Could you check a few things on this drawing? It's one solid part, dimensions in mm from its lowest x, y, z. A direction names the side the tool comes from. Round coordinates to 2 decimals unless told otherwise and drop trailing zeros. Loops run counter-clockwise (first coordinate to the right, second up) from the corner with the lowest first, then second, coordinate; pieces in that order, holes last. Notation, with made-up numbers: M 10,75.5 L 66,75.5 A11 cw 66,91.5 Z; hole C -37,-34 d2. An arc over 180 degrees is marked long. Put each result on its own line as item: value. Start each with the question number.
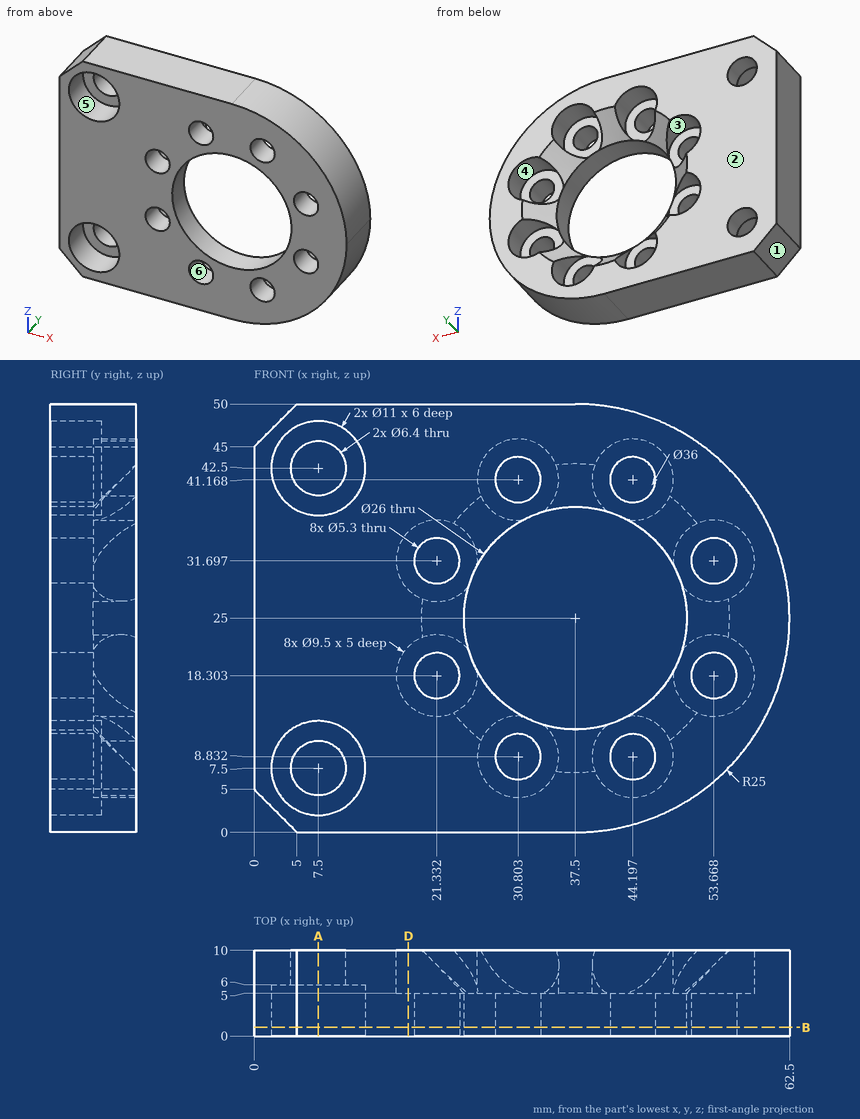
1) Suppose I cut it at B-B (y = 1). State how many separate pieces and enclosed holes the cut face has, plus the area to 3 significant figures.
2) If I drill on probe 1 along Z at (x, y) = (43.5, 4) (1 decimal); probe 2 along X at (y, z) = (1.25, 42); probe 3 along Z at (x, y) = (4.5, 4.75), over which ranges is the centre line in solid material (lowest first)? Write a range as from..to.
3) If we mould it in two halves opening along Z, with no side actions, what happens to the marked faces 1, 2 and 3? For each: pulls with the +Z half, pulls with the -Z half, needs draft (parallel to the pull), parting line crosses it, or undercut.
4) Suppose I cut it at D-D (x = 18). Write out the boundary of the cut face in (y, z).
5) On a 3-axis mill with a long thin cutter (end or side, diameter ignored), from which of +Z, -Z, +X, -X, +Y, -Y can I reach the whole of each face in a straight line? I mean the marked faces 4, 5 and 6. Say none if no direction works.
6) Suppose I cut it at A-A (x = 7.5). Write out the boundary of the cut face in (y, z).
7) I'm going to push flat-ended pins straight in: P1, Ø4.5, axis at x = 33, z = 8, coming from the +Y side; P2, Ø3, axis at x = 44.2, z = 41.17, coming from the +Y side; P3, Ø1.5, axis at y = 4, z = 37, coming from the +X side; P4, Ø1, axis at y = 3, z = 9.5, coming from the +X side. Where does each tip first touch, or does it pass through?
Results are:
1. separate pieces: 1
1. enclosed holes: 11
1. area: 1,930 mm²
2. probe 1: 0.7..6.3, 11.4..13.5, 36.5..38.6, 43.7..49.3
2. probe 2: 0..2.02, 12.98..28.29, 33.32..41.68, 46.71..55.83
2. probe 3: 0.5..2.89, 12.11..37.89, 47.11..49.5
3. face 1: pulls with the -Z half
3. face 2: needs draft
3. face 3: undercut
4. outline: M 0,0 L 10,0 L 10,14.92 L 5,14.92 L 5,21.69 L 10,21.69 L 10,28.31 L 5,28.31 L 5,35.08 L 10,35.08 L 10,50 L 0,50 Z
5. face 4: +Y
5. face 5: -Y
5. face 6: +Y, -Y
6. outline: M 0,0 L 10,0 L 10,4.3 L 6,4.3 L 6,2 L 0,2 Z; M 0,13 L 6,13 L 6,10.7 L 10,10.7 L 10,39.3 L 6,39.3 L 6,37 L 0,37 Z; M 0,48 L 6,48 L 6,45.7 L 10,45.7 L 10,50 L 0,50 Z
7. P1: y = 5
7. P2: through
7. P3: x = 59.83
7. P4: x = 57.5
